```python
from build123d import *

# Parameters (mm, degrees)
SKETCH1_W           = 98
SKETCH1_H           = 8
BOSS_EXTRUDE1_DEPTH = 265
CUT_EXTRUDE2_DEPTH  = 265


with BuildPart() as part:
    # Sketch1 → Boss-Extrude1 (new body)
    with BuildSketch(Plane.XY):
        with Locations((49, 4)):
            Rectangle(SKETCH1_W, SKETCH1_H)
    extrude(amount=-BOSS_EXTRUDE1_DEPTH)

    # Sketch2 → Cut-Extrude2 (cut)
    with BuildSketch(Plane.XY):
        Polygon((2.245049024, 8), (1.195049024, 2.75), (6.804950976, 2.75), (5.754950976, 8), align=None)
    extrude(amount=-CUT_EXTRUDE2_DEPTH, mode=Mode.SUBTRACT)


solid = part.part
```
CAD build for the part. Positions are in the model's coordinates, mm. A direction names the side the tool comes from. Round coordinates to 2 decimals unless told otherwise and drop trailing zeros. Loops run counter-clockwise (first coordinate to the right, second up) from the corner with the lowest first, then second, coordinate; pieces in that order, holes last. Notation, with made-up numbers: M 27.25,62 L 40.25,62 A36 cw 40.25,98 Z; hole C -17.75,75.25 d8. An arc over 180 degrees is marked long. Use a Markdown table: item, result. Add a question column.
(1) Which spindle directions (+Z, -Z, +X, -X, +Y, -Y) get a long thin tool onto all of the face, cutting with end or side? Do faces 4 (the face through (4, 2.75, -131)), 5 (the face through (48, 4, -265)). Say none if no direction does.
(2) Cut at B-B (z = -23). Give the cut face in (x, y).
(3) Cut at A-A (y = 6.25). Give the cut face in (x, z).
(4) Drill centre lines: line 1 (X direction, y = 3, z = -118); line 2 (X direction, y = 7.75, z = -215). Where is each one in solid material? Low to high.
(5) Pull direction X, two halves, no side cores. Call faces 1 (the face through (48, 4, 0)), 2 (the face through (98, 4, -131)), 3 (the face through (1.727, 5.412, -130.645)): +X half, -X half, draft (parallel to the pull), parting line (faces both ways), or undercut.
Geometry says:
| question | item | result |
|---|---|---|
| 1 | face 4 | +Z, -Z |
| 1 | face 5 | -Z, +X, -X, +Y, -Y |
| 2 | outline | M 0,0 L 98,0 L 98,8 L 5.75,8 L 6.8,2.75 L 1.2,2.75 L 2.25,8 L 0,8 Z |
| 3 | outline | M 0,-265 L 1.9,-265 L 1.9,0 L 0,0 Z; M 6.1,-265 L 98,-265 L 98,0 L 6.1,0 Z |
| 4 | line 1 | x = 0 to 1.25, 6.75 to 98 |
| 4 | line 2 | x = 0 to 2.2, 5.8 to 98 |
| 5 | face 1 | draft |
| 5 | face 2 | +X half |
| 5 | face 3 | undercut |
